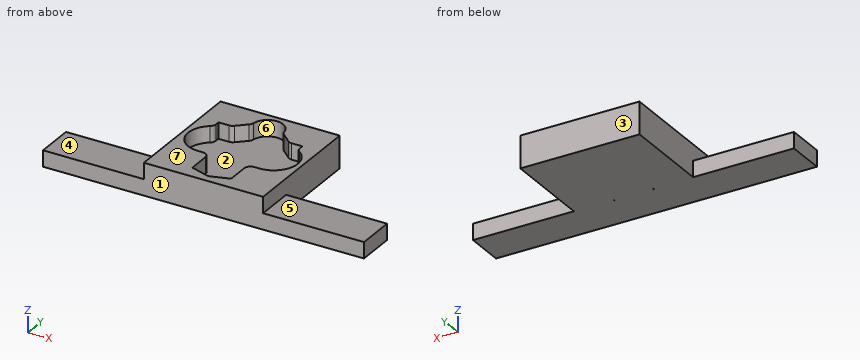
from build123d import *

# Parameters (mm, degrees)
F1_W     = 37.15
F1_H     = 39.9213461205
F2_DEPTH = 5
F3_R     = 2
F4_W     = 31.425
F4_H     = 12
F5_DEPTH = 5
F7_DEPTH = 5


with BuildPart() as f2:
    # F1 (on Top) → F2 (new body)
    with BuildSketch(Plane.XY):
        with Locations((17.075, 17.5686092116)):
            Rectangle(F1_W, F1_H)
        with BuildLine():
            ThreePointArc((7.475, 10.7), (0.2160219573, 16.3909420481), (4.01, 24.7983979195))
            Line((4.01, 24.7983979195), (4.01, 27.23))
            Line((4.01, 27.23), (8.075, 27.23))
            Line((8.075, 27.23), (12.255, 30.99))
            ThreePointArc((12.255, 30.99), (17.075, 35.81), (21.895, 30.99))
            Line((21.895, 30.99), (26.075, 27.23))
            Line((26.075, 27.23), (30.14, 27.23))
            Line((30.14, 27.23), (30.14, 24.7983979195))
            ThreePointArc((30.14, 24.7983979195), (33.9339780427, 16.3909420481), (26.675, 10.7))
            Line((26.675, 10.7), (23.11, 10.7))
            Line((23.11, 10.7), (23.11, 1.9))
            Line((23.11, 1.9), (17.075, 0))
            Line((17.075, 0), (11.04, 1.9))
            Line((11.04, 1.9), (11.04, 10.7))
            Line((11.04, 10.7), (7.475, 10.7))
        make_face(mode=Mode.SUBTRACT)
    extrude(amount=F2_DEPTH)

    # F3
    f3_edges = [f2.edges().sort_by_distance(p)[0] for p in [
        (8.075, 27.23, 2.5),
        (12.255, 30.99, 2.5),
        (21.895, 30.99, 2.5),
        (26.075, 27.23, 2.5),
        (30.14, 24.798398, 2.5),
        (4.01, 24.798398, 2.5),
        (11.04, 10.7, 2.5),
        (23.11, 10.7, 2.5),
    ]]
    fillet(f3_edges, radius=F3_R)

    # F4 (on face) + F0 (on Top) → F5 (join)
    with BuildSketch(Plane(origin=(0, 0, 0), x_dir=(1, 0, 0), z_dir=(0, 0, -1))):
        with Locations((-17.2125, -3.6079361513)):
            Rectangle(F4_W, F4_H)
        with Locations((51.3625, -3.6079361513)):
            Rectangle(F4_W, F4_H)
        with BuildLine():
            Line((23.3279641011, -9.6079361513), (35.65, -9.6079361513))
            Line((35.65, -9.6079361513), (35.65, 2.3920638487))
            Line((35.65, 2.3920638487), (-1.5, 2.3920638487))
            Line((-1.5, 2.3920638487), (-1.5, -9.6079361513))
            Line((-1.5, -9.6079361513), (10.8220358989, -9.6079361513))
            ThreePointArc((10.8220358989, -9.6079361513), (10.9847457158, -9.1668662561), (11.04, -8.7))
            Line((11.04, -8.7), (11.04, -1.9))
            Line((11.04, -1.9), (17.075, 0))
            Line((17.075, 0), (23.11, -1.9))
            Line((23.11, -1.9), (23.11, -8.7))
            ThreePointArc((23.11, -8.7), (23.1652542842, -9.1668662561), (23.3279641011, -9.6079361513))
        make_face()
    with BuildSketch(Plane.XY):
        Polygon((11.04, 1.9), (17.075, 0), (17.075, 10.7), (11.04, 10.7), align=None)
        Polygon((17.075, 10.7), (17.075, 0), (23.11, 1.9), (23.11, 10.7), align=None)
    extrude(amount=F5_DEPTH, dir=(0, 0, -1))

    # F6 (on face) → F7 (join)
    with BuildSketch(Plane(origin=(0, 0, 0), x_dir=(1, 0, 0), z_dir=(0, 0, -1))):
        with BuildLine():
            Line((-1.5, -37.5292822719), (35.65, -37.5292822719))
            Line((35.65, -37.5292822719), (35.65, -9.6079361513))
            Line((35.65, -9.6079361513), (23.3279641011, -9.6079361513))
            ThreePointArc((23.3279641011, -9.6079361513), (24.0649814123, -10.4052671789), (25.11, -10.7))
            Line((25.11, -10.7), (26.675, -10.7))
            ThreePointArc((26.675, -10.7), (33.7996177752, -15.9132647022), (30.9864379947, -24.2813186469))
            ThreePointArc((30.9864379947, -24.2813186469), (30.3641728673, -24.9950956291), (30.14, -25.9151162782))
            Line((30.14, -25.9151162782), (30.14, -27.23))
            Line((30.14, -27.23), (26.8421686802, -27.23))
            ThreePointArc((26.8421686802, -27.23), (26.125888011, -27.3626644643), (25.504632333, -27.7430579971))
            Line((25.504632333, -27.7430579971), (22.4908367694, -30.4540319969))
            ThreePointArc((22.4908367694, -30.4540319969), (22.0628330313, -31.0013633318), (21.8479117921, -31.662095994))
            ThreePointArc((21.8479117921, -31.662095994), (17.075, -35.81), (12.3020882079, -31.662095994))
            ThreePointArc((12.3020882079, -31.662095994), (12.0871669687, -31.0013633318), (11.6591632306, -30.4540319969))
            Line((11.6591632306, -30.4540319969), (8.645367667, -27.7430579971))
            ThreePointArc((8.645367667, -27.7430579971), (8.024111989, -27.3626644643), (7.3078313198, -27.23))
            Line((7.3078313198, -27.23), (4.01, -27.23))
            Line((4.01, -27.23), (4.01, -25.9151162782))
            ThreePointArc((4.01, -25.9151162782), (3.7858271327, -24.9950956291), (3.1635620053, -24.2813186469))
            ThreePointArc((3.1635620053, -24.2813186469), (0.3503822248, -15.9132647022), (7.475, -10.7))
            Line((7.475, -10.7), (9.04, -10.7))
            ThreePointArc((9.04, -10.7), (10.0850185877, -10.4052671789), (10.8220358989, -9.6079361513))
            Line((10.8220358989, -9.6079361513), (-1.5, -9.6079361513))
            Line((-1.5, -9.6079361513), (-1.5, -37.5292822719))
        make_face()
        with BuildLine():
            ThreePointArc((25.11, -10.7), (24.0649814123, -10.4052671789), (23.3279641011, -9.6079361513))
            Line((23.3279641011, -9.6079361513), (10.8220358989, -9.6079361513))
            ThreePointArc((10.8220358989, -9.6079361513), (10.0850185877, -10.4052671789), (9.04, -10.7))
            Line((9.04, -10.7), (7.475, -10.7))
            ThreePointArc((7.475, -10.7), (0.3503822248, -15.9132647022), (3.1635620053, -24.2813186469))
            ThreePointArc((3.1635620053, -24.2813186469), (3.7858271327, -24.9950956291), (4.01, -25.9151162782))
            Line((4.01, -25.9151162782), (4.01, -27.23))
            Line((4.01, -27.23), (7.3078313198, -27.23))
            ThreePointArc((7.3078313198, -27.23), (8.024111989, -27.3626644643), (8.645367667, -27.7430579971))
            Line((8.645367667, -27.7430579971), (11.6591632306, -30.4540319969))
            ThreePointArc((11.6591632306, -30.4540319969), (12.0871669687, -31.0013633318), (12.3020882079, -31.662095994))
            ThreePointArc((12.3020882079, -31.662095994), (17.075, -35.81), (21.8479117921, -31.662095994))
            ThreePointArc((21.8479117921, -31.662095994), (22.0628330313, -31.0013633318), (22.4908367694, -30.4540319969))
            Line((22.4908367694, -30.4540319969), (25.504632333, -27.7430579971))
            ThreePointArc((25.504632333, -27.7430579971), (26.125888011, -27.3626644643), (26.8421686802, -27.23))
            Line((26.8421686802, -27.23), (30.14, -27.23))
            Line((30.14, -27.23), (30.14, -25.9151162782))
            ThreePointArc((30.14, -25.9151162782), (30.3641728673, -24.9950956291), (30.9864379947, -24.2813186469))
            ThreePointArc((30.9864379947, -24.2813186469), (33.7996177752, -15.9132647022), (26.675, -10.7))
            Line((26.675, -10.7), (25.11, -10.7))
        make_face()
    extrude(amount=F7_DEPTH)


solid = f2.part
CAD build for the part. Positions are in the model's coordinates, mm. Face numbers are marked on the shaded views. A direction names the side the tool comes from. Round coordinates to 2 decimals unless told otherwise and drop trailing zeros. Write each loop counter-clockwise with the first axis right and the second up, starting at its lowest first coordinate (ties: lowest second). Pieces come first, ordered by that corner, then holes.
(1) Slice it at D-D, the plane x = -18. Write the cut outline in (y, z).
(2) Slice it at C-C, the plane z = -2.25. Write the cut outline in (x, y) (3 decimals).
(3) Slice it at A-A, the plane z = 2. Write the cut outline in (x, y) (3 decimals), and give its area (3 significant figures).
(4) Slice it at B-B, the plane y = 5. Write the cut outline in (x, z) (3 decimals).
(5) Drop flat-ended pins along their axis: P1, Ø6, axis at x = -14, y = 2.5, coming from the +Z side; P2, Ø1.5, axis at y = 4.5, z = 3.5, coming from the +X side; P3, Ø10, axis at x = 14, y = 12.5, coming from the +Z side; P4, Ø0.7, axis at y = 27, z = 2.5, coming from the -X side. Give the stop position or say it passes through.
(6) 3-axis set-ups, long thin cutter, end or side, ignore diameter. For the marked faces 5, 6 and 7: which of +Z, -Z, +X, -X, +Y, -Y reach the whole face in a straight line?
(7) Mould opens along Y. For the marked faces 1, 2, 3 and 4 say: pulls with the +Y half, pulls with the -Y half, needs draft (parallel to the pull), parting line crosses it, or undercut.
(8) Probe line 1 along Y through (x, z) = (7, 2); line 2 along X through (y, z) = (2, 2.5); line 3 along X through (y, z) = (36, -1.75). List the from-to ranges inside material, lowest first.
From the geometry:
1. outline: (-2.39, -5) - (9.61, -5) - (9.61, 0) - (-2.39, 0) - close
2. outline: (-32.925, -2.392) - (67.075, -2.392) - (67.075, 9.608) - (35.65, 9.608) - (35.65, 37.529) - (-1.5, 37.529) - (-1.5, 9.608) - (-32.925, 9.608) - close; hole (10.822, 9.608) arc R2 cw to (11.04, 8.7) - (11.04, 9.608) - close; hole (23.11, 8.7) arc R2 cw to (23.328, 9.608) - (23.11, 9.608) - close
3. outline: (-1.5, -2.392) - (35.65, -2.392) - (35.65, 37.529) - (-1.5, 37.529) - close; hole (3.164, 24.281) arc R7.475 ccw to (7.475, 10.7) - (9.04, 10.7) arc R2 cw to (11.04, 8.7) - (11.04, 1.9) - (17.075, 0) - (23.11, 1.9) - (23.11, 8.7) arc R2 cw to (25.11, 10.7) - (26.675, 10.7) arc R7.475 ccw to (30.986, 24.281) arc R2 cw to (30.14, 25.915) - (30.14, 27.23) - (26.842, 27.23) arc R2 cw to (25.505, 27.743) - (22.491, 30.454) arc R2 cw to (21.848, 31.662) arc R4.82 ccw to (12.302, 31.662) arc R2 cw to (11.659, 30.454) - (8.645, 27.743) arc R2 cw to (7.308, 27.23) - (4.01, 27.23) - (4.01, 25.915) arc R2 cw to start
3. area: 769 mm2
4. outline: (-32.925, -5) - (67.075, -5) - (67.075, 0) - (35.65, 0) - (35.65, 5) - (23.11, 5) - (23.11, 0) - (11.04, 0) - (11.04, 5) - (-1.5, 5) - (-1.5, 0) - (-32.925, 0) - close
5. P1: stops at z = 0
5. P2: stops at x = 35.65
5. P3: stops at z = 5
5. P4: stops at x = -1.5
6. face 5: +Z, +X, +Y, -Y
6. face 6: +Z
6. face 7: +Z, +X, -X, +Y, -Y
7. face 1: pulls with the -Y half
7. face 2: undercut
7. face 3: pulls with the +Y half
7. face 4: needs draft
8. line 1: y = -2.39 to 10.72, 27.23 to 37.53
8. line 2: x = -1.5 to 11.04, 23.11 to 35.65
8. line 3: x = -1.5 to 35.65
